Check sheet for the modelled part. Datum: model origin and axes. Units: mm. A direction names the side the tool comes from. Give positions to 0.01 mm unless a question says otherwise; leave off trailing zeros. Write each loop counter-clockwise with the first axis right and the second up, starting at its lowest first coordinate (ties: lowest second). Pieces come first, ordered by that corner, then holes. Notation, with made-up numbers: M 88,58.5 L 127,58.5 A25 ccw 127,90.5 Z; hole C 8,-19.5 d8. An arc over 180 degrees is marked long. Use CSV: the item, a comma, the result in double quotes. Start each with the question number.
1. Cross-section at C-C, the plane z = 5.75. Enter the section's corners in (x, y), and give its area (3 significant figures).
2. Scan lines: line 1 (X direction, y = 0.5, z = 2.25); line 2 (Z direction, x = 2.75, y = 5.25); line 3 (X direction, y = 3.5, z = 3). Record each from-to range of solid material in increasing order.
3. Cross-section at B-B, the plane x = -9.5. Enter the section's corners in (y, z), and give its area (3 significant figures).
4. Access from +Z, -Z, +X, -X, +Y, -Y to the whole of each face (thin tool, end or side, straight path). Record for faces 5 (the face through (8, 4.565, 2)), 6 (the face through (0, 5, 0)), 7 (the face through (0, 3.565, -1)).
5. Mould release check, pull along X, two halves, no side actions. Record for faces 1 (the face through (13.439, 2, 3)), 2 (the face through (-10, 2, 0)), 3 (the face through (-9.34, 2.31, 1.43)), 4 (the face through (0, 5, 6)): +X half, -X half, draft (parallel to the pull), parting line (faces both ways), or undercut.
6. Cross-section at A-A, the plane z = 3. Enter the section's corners in (x, y), and give its area (3 significant figures).
7. Cross-section at D-D, the plane y = 5. Enter the section's corners in (x, z), and give its area (3 significant figures).
8. Depth check by flat-ended pin: P1, Ø3, axis at x = 10.01, z = 3, coming from the +Y side; P2, Ø5, axis at x = -2.5, z = 3.5, coming from the -Y side; P3, Ø3.5, axis at x = -7.5, y = 2, coming from the -Z side; P4, Ø0.6, axis at x = 2.5, z = 7, coming from the -Y side. Enter the tip coordinate at first touch or a pass-through.
Autodesk Inventor part; units mm, degrees
ref_plane "YZ Plane" through (0, 0, 0) normal (1, 0, 0) x (0, 1, 0)
ref_plane "XZ Plane" through (0, 0, 0) normal (0, 1, 0) x (-1, 0, 0)
ref_plane "XY Plane" through (0, 0, 0) normal (0, 0, 1) x (1, 0, 0)
sketch "Sketch1" plane through (0, 0, 0) normal (0, 0, 1) x (1, 0, 0)
  line L0 (0, 0) -> (-6.4135, 0)
  line L1 (-6.4135, 0) -> (-3.2004, 5.5653)
  line L2 (-3.2004, 5.5653) -> (3.2258, 5.5653)
  line L3 (3.2258, 5.5653) -> (6.4389, 0)
  line L4 (6.4389, 0) -> (3.2258, -5.5653)
  line L5 (3.2258, -5.5653) -> (-3.2004, -5.5653)
  line L6 (-3.2004, -5.5653) -> (-6.4135, 0)
  line L7 (-6.4135, 0) -> (-13.4135, 0)
  line L8 (-6.4135, 0) -> (0.5865, 0) construction
  line L9 (-13.4135, 0) -> (-13.4135, 5.5653)
  line L10 (-13.4135, 5.5653) -> (-13.4135, 9.5653)
  line L11 (-13.4135, 9.5653) -> (13.4389, 9.5653)
  line L12 (13.4389, 9.5653) -> (13.4389, 0)
  line L13 (13.4389, 0) -> (6.4389, 0)
  line L14 (13.4389, 9.5653) -> (13.4389, 4.5653)
  line L15 (13.4389, 4.5653) -> (6.4389, 4.5653)
  line L16 (6.4389, 4.5653) -> (6.4389, 9.5653)
  line L17 (-13.4135, 9.5653) -> (-6.4135, 9.5653)
  line L18 (-6.4135, 9.5653) -> (-6.4135, 4.5653)
  line L19 (-6.4135, 4.5653) -> (-13.4135, 4.5653)
  dimension "d0" = 6.4135
  dimension "d1" = 6.4262
  dimension "d2" = 60
  dimension "d3" = 6.4262
  dimension "d4" = 120
  dimension "d5" = 6.4262
  dimension "d6" = 120
  dimension "d7" = 6.4262
  dimension "d8" = 120
  dimension "d9" = 6.4262
  dimension "d10" = 120
  dimension "d11" = 7
  dimension "d12" = 180
  dimension "d13" = 4
  dimension "d15" = 5
  dimension "d16" = 7
  dimension "d17" = 7
  dimension "d20" = 7
extrude "Extrusion1" add sketch "Sketch1" along normal blind 6 contours L7 L9 L19 L18 L11 L16 L15 L12 L13 L3 L2 L1
sketch "Sketch3" plane through (0, 0, 0) normal (0, 0, -1) x (-1, 0, 0)
  line L0 (-6.4389, 4.5653) -> (-6.4389, 9.5653)
  line L1 (-6.4389, 9.5653) -> (-6.4389, 3.5653)
  line L2 (-6.4389, 3.5653) -> (6.4135, 3.5653)
  line L3 (6.4135, 9.5653) -> (6.4135, 4.5653)
  line L4 (-6.4389, 9.5653) -> (6.4135, 9.5653)
  line L5 (6.4135, 3.5653) -> (6.4135, 9.5653)
  line L6 (6.4135, 9.5653) -> (-6.4389, 9.5653)
  point P0 (0, 0)
  point P1 (6.4135, 4.5653)
  point P2 (-6.4389, 4.5653)
  dimension "d30" = 6
extrude "Extrusion2" add sketch "Sketch3" along normal blind 2
sketch "Sketch4" plane through (-13.4135, 0, 0) normal (0, -1, 0) x (1, 0, 0)
  line L0 (0, 0) -> (0, 6)
  line L1 (0, 3) -> (26.8524, 3)
  line L2 (26.8524, 0) -> (26.8524, 6)
  line L3 (13.4262, 3) -> (3.4262, 3)
  line L4 (3.4262, 3) -> (23.4262, 3)
  point P0 (13.4135, 0)
  dimension "d36" = 10
  dimension "d37" = 20
  dimension "d38" = 0
hole "Hole2" at (-9.9873, 0, 3) at (10.0127, 0, 3) direction (0, 1, 0) diameter 3.4 end through all
sketch "Sketch5" plane through (-6.4135, 9.5653, 6) normal (0, 1, 0) x (1, 0, 0)
  line L0 (12.8524, 6) -> (12.8524, 0)
  line L1 (12.8524, 0) -> (0, 0)
  line L2 (0, 0) -> (0, -2)
  line L3 (0, -2) -> (12.8524, -2)
  line L4 (12.8524, -2) -> (12.8524, 0)
  point P0 (6.4135, 6)
  dimension "d46" = 2
extrude "Extrusion3" add sketch "Sketch5" against normal blind 5
properties part number "shell 1.0 screw top"
Worked answers:
1,outline,"M -13.41,0 L -6.41,0 L -3.2,5.57 L 3.23,5.57 L 6.44,0 L 13.44,0 L 13.44,4.57 L 6.44,4.57 L 6.44,9.57 L -6.41,9.57 L -6.41,4.57 L -13.41,4.57 Z"
1,area,"133 mm^2"
2,line 1,"x = -13.41 to -11.51, -8.46 to -6.12, 6.15 to 8.49, 11.54 to 13.44"
2,line 2,"z = -2 to 0, 6 to 8"
2,line 3,"x = -13.41 to -11.69, -8.29 to -4.39, 4.42 to 8.31, 11.71 to 13.44"
3,outline,"M 0,0 L 4.57,0 L 4.57,1.37 L 0,1.37 Z; M 0,4.63 L 4.57,4.63 L 4.57,6 L 0,6 Z"
3,area,"12.5 mm^2"
4,face 5,"+Z, -Z, +X, +Y"
4,face 6,"-Y"
4,face 7,"-Z, +X, -X, -Y"
5,face 1,"+X half"
5,face 2,"draft"
5,face 3,"undercut"
5,face 4,"undercut"
6,outline,"M -13.41,0 L -11.69,0 L -11.69,4.57 L -13.41,4.57 Z; M -8.29,0 L -6.41,0 L -3.2,5.57 L 3.23,5.57 L 6.44,0 L 8.31,0 L 8.31,4.57 L 6.44,4.57 L 6.44,9.57 L -6.41,9.57 L -6.41,4.57 L -8.29,4.57 Z; M 11.71,0 L 13.44,0 L 13.44,4.57 L 11.71,4.57 Z"
6,area,"102 mm^2"
7,outline,"M -6.41,-2 L 6.44,-2 L 6.44,8 L -6.41,8 Z; hole M -3.53,0 L 3.55,0 L 3.55,6 L -3.53,6 Z"
7,area,"86.1 mm^2"
8,P1,"passes through"
8,P2,"stops at y = 2.45"
8,P3,"stops at z = 0"
8,P4,"stops at y = 4.57"
